Verification items for this drawing (mm, ordinates from the low corner). Round coordinates to 2 decimals unless told otherwise and drop trailing zeros. Order: outer loops, then holes, each group sorted by start corner. A loop starts at its lowest first (then second) coordinate and runs counter-clockwise, first axis right, second up. Notation, with made-up numbers: (7, 47) -> (24, 47) arc R36 cw to (24, 86) -> close; hole circle Ø9 at (53.25, 35). An arc over 180 degrees is marked (long way). Return JSON: item names as keys, results as strings. Group by question number.
Item 1: Scan lines: probe 1 along X at (y, z) = (5, 4); probe 2 along Z at (x, y) = (157.5, 9.5); probe 3 along Z at (x, y) = (74.5, 7.5). Record each from-to range of solid material in increasing order. Write a range as from..to.
Item 2: Sectioned sample at A-A on z = 25. Record the cut outline in (x, y), plus the area to 3 significant figures.
Item 3: Depth check by flat-ended pin: pin 1 Ø8 at (x, z) = (59.5, 33) entering from -Y; pin 2 Ø5 at (x, y) = (156, 4) entering from -Z; pin 3 Ø1.5 at (x, y) = (24.5, 1.5) entering from -Z; pin 4 Ø1.5 at (x, y) = (121, 4) entering from -Z. Enter the tip coordinate at first touch or a pass-through.
Item 4: Sectioned sample at D-D on x = 156.5. Record the cut outline in (y, z), plus the area to 3 significant figures.
Item 5: Sectioned sample at C-C on y = 3.5. Record the cut outline in (x, z).
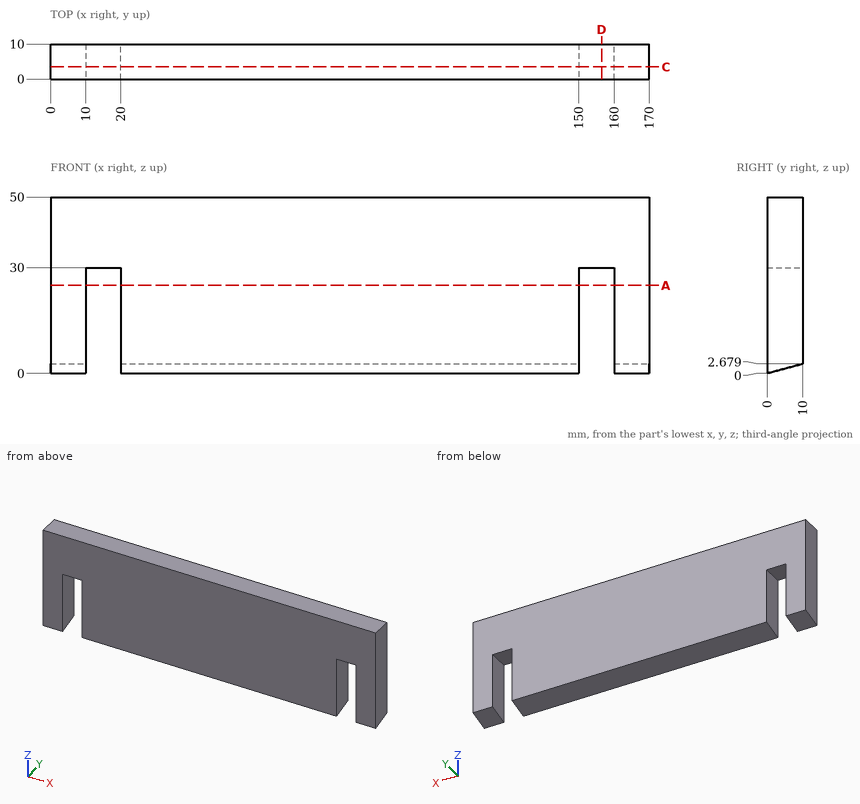
Recorded:
{
 "1": {"probe 1": "0..10, 20..150, 160..170", "probe 2": "30..50", "probe 3": "2.01..50"},
 "2": {"outline": "(0, 0) -> (10, 0) -> (10, 10) -> (0, 10) -> close; (20, 0) -> (150, 0) -> (150, 10) -> (20, 10) -> close; (160, 0) -> (170, 0) -> (170, 10) -> (160, 10) -> close", "area": "1,500 mm²"},
 "3": {"pin 1": "y = 0", "pin 2": "z = 30", "pin 3": "z = 0.2", "pin 4": "z = 0.87"},
 "4": {"outline": "(0, 30) -> (10, 30) -> (10, 50) -> (0, 50) -> close", "area": "200 mm²"},
 "5": {"outline": "(0, 0.94) -> (10, 0.94) -> (10, 30) -> (20, 30) -> (20, 0.94) -> (150, 0.94) -> (150, 30) -> (160, 30) -> (160, 0.94) -> (170, 0.94) -> (170, 50) -> (0, 50) -> close"}
}
